Geometry: final body of the model. Coordinates: model frame, mm. Face numbers are marked on the shaded views. A direction names the side the tool comes from. Give positions to 0.01 mm unless a question says otherwise; leave off trailing zeros. Write each loop counter-clockwise with the first axis right and the second up, starting at its lowest first coordinate (ties: lowest second). Pieces come first, ordered by that corner, then holes. Notation, with made-up numbers: M 54.25,-37.75 L 93.25,-37.75 A33 ccw 93.25,-9.75 Z; hole C 18,-30 d2. An arc over 180 degrees is marked long. Use one line per item in the form item = value. Start each with the question number.
Item 1: Section query A-A on y = 0. Return loops of the section in (x, z), then the cut area to 3 significant figures.
Item 2: Section query B-B on x = 0. Return loops of the section in (y, z).
Item 3: Pull-direction query (Y, two-part tool) for the marked faces 1, 2 and 3; classes: released by +Y, released by -Y, zero draft, split by the parting line, or undercut.
Item 4: Material intervals for line 1 along Y through (x, z) = (0, 12.45); line 2 along Z through (x, y) = (1.25, 1.25); line 3 along Y through (x, z) = (0, 5.5), sorted ascending. Write a range as from..to.
Item 5: Section query C-C on z = 6.5. Return loops of the section in (x, y), then the cut area to 3 significant figures.
Item 6: Section query D-D on x = -7. Return loops of the section in (y, z), then the cut area to 3 significant figures.
Item 7: Contact query for flat-ended pins moving along their axis: P1, Ø3.5, axis at x = -4.5, z = 3.5, coming from the -Y side; P2, Ø1.5, axis at y = -4, z = 1.5, coming from the -X side; P3, Ø4, axis at x = -3.5, z = 2.5, coming from the +Y side. Output: stop coordinate, or through.
Item 8: Access query for the marked faces 4, 5 and 6. Directions: +Z, -Z, +X, -X, +Y, -Y. A direction counts if a zero-diameter tool reaches every point of the face in a straight line with its end or side. Return the directions, or none.
from build123d import *

# Parameters (mm, degrees)
SKETCH136_R     = 9
PAD081_DEPTH    = 13
POCKET045_DEPTH = 8
SKETCH138_R     = 3.1
POCKET046_DEPTH = 2.6
SKETCH139_R     = 1.75
POCKET047_DEPTH = 9.001


with BuildPart() as part:
    # Sketch136 → Pad081 (new body)
    with BuildSketch(Plane.XY):
        Circle(SKETCH136_R)
    extrude(amount=PAD081_DEPTH)

    # Sketch137 → Pocket045 (cut)
    with BuildSketch(Plane.XY):
        with BuildLine():
            Line((-3.152776, 2.850001), (-6.25, 2.850001))
            Line((-6.25, 2.850001), (-6.25, -2.850001))
            Line((-6.25, -2.850001), (-3.152776, -2.850001))
            ThreePointArc((-3.152776, -2.850001), (4.25, 0), (-3.152776, 2.850001))
        make_face()
    extrude(amount=POCKET045_DEPTH, mode=Mode.SUBTRACT)

    # Sketch138 → Pocket046 (cut)
    with BuildSketch(Plane.XY.offset(13)):
        Circle(SKETCH138_R)
    extrude(amount=-POCKET046_DEPTH, mode=Mode.SUBTRACT)

    # Sketch139 → Pocket047 (cut, through all)
    with BuildSketch(Plane.YZ):
        with Locations((0, 4)):
            Circle(SKETCH139_R)
    extrude(amount=-POCKET047_DEPTH, mode=Mode.SUBTRACT)


solid = part.part
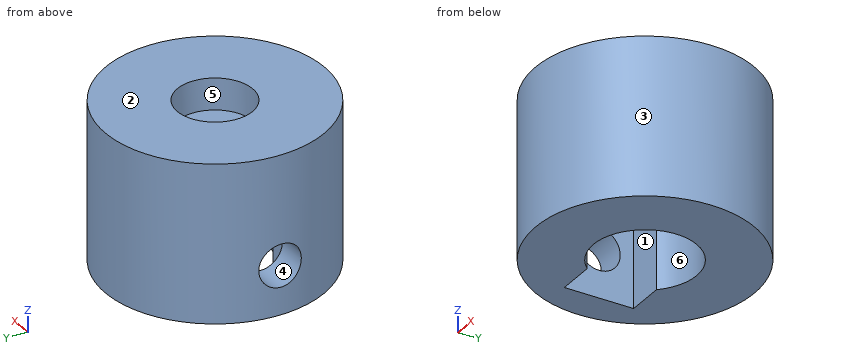
Answer sheet:
q1.outline = M -9,0 L -6.25,0 L -6.25,2.25 L -9,2.25 Z; M -9,5.75 L -6.25,5.75 L -6.25,8 L 4.25,8 L 4.25,0 L 9,0 L 9,13 L 3.1,13 L 3.1,10.4 L -3.1,10.4 L -3.1,13 L -9,13 Z
q1.area = 124 mm2
q2.outline = M -9,0 L -4.25,0 L -4.25,8 L 4.25,8 L 4.25,0 L 9,0 L 9,13 L 3.1,13 L 3.1,10.4 L -3.1,10.4 L -3.1,13 L -9,13 Z
q3.face_1 = undercut
q3.face_2 = zero draft
q3.face_3 = split by the parting line
q4.line_1 = -9..-3.1, 3.1..9
q4.line_2 = 8..10.4
q4.line_3 = -9..-4.25, 4.25..9
q5.outline = C 0,0 d18; hole M -6.25,-2.85 L -3.15,-2.85 A4.25 ccw long -3.15,2.85 L -6.25,2.85 Z
q5.area = 184 mm2
q6.outline = M -5.66,0 L 5.66,0 L 5.66,13 L -5.66,13 Z; hole C 0,4 d3.5
q6.area = 137 mm2
q7.P1 = -8.57
q7.P2 = -8.39
q7.P3 = 8.87
q8.face_4 = -X
q8.face_5 = +Z
q8.face_6 = -Z
